Geometry check sheet. Reference: the model listing, model coordinates, mm. A direction names the side the tool comes from. Give positions to 0.01 mm unless a question says otherwise; leave off trailing zeros. Write each loop counter-clockwise with the first axis right and the second up, starting at its lowest first coordinate (ties: lowest second). Pieces come first, ordered by that corner, then holes. Notation, with made-up numbers: (12, 26.25) -> (42, 26.25) arc R20 cw to (42, 35.25) -> close; hole circle Ø4 at (-7, 3). An arc over 180 degrees is marked (long way). Use a Markdown table: item, result. Add a question column.
from build123d import *

# Parameters (mm, degrees)
SKETCH_1_R          = 3
EXTRUDE_1_DEPTH     = 18
CHAMFER_1_SIZE      = 0.5
CUT_EXTRUDE_1_DEPTH = 12


with BuildPart() as part:
    # Эскиз1 → Бобышка-Вытянуть1 (new body)
    with BuildSketch(Plane(origin=(0, 0, 0), x_dir=(1, 0, 0), z_dir=(0, 1, 0))):
        Circle(SKETCH_1_R)
    extrude(amount=EXTRUDE_1_DEPTH)

    # Фаска1
    chamfer_1_edges = [part.edges().sort_by_distance(p)[0] for p in [
        (-3, 18, 0),
    ]]
    chamfer(chamfer_1_edges, length=CHAMFER_1_SIZE)

    # Эскиз2 → Вырез-Вытянуть1 (cut)
    with BuildSketch(Plane(origin=(0, 18, 0), x_dir=(1, 0, 0), z_dir=(0, 1, 0))):
        with BuildLine():
            Line((-2.4, 1.8), (2.4, 1.8))
            ThreePointArc((2.4, 1.8), (0, 3), (-2.4, 1.8))
        make_face()
    extrude(amount=-CUT_EXTRUDE_1_DEPTH, mode=Mode.SUBTRACT)


solid = part.part
1) Sectioned sample at A-A, the plane x = 0. Enter the section's corners in (y, z), and give its area (3 significant figures).
2) Sectioned sample at D-D, the plane y = 8.5. Enter the section's corners in (x, z).
3) Sectioned sample at C-C, the plane z = -2.45. Enter the section's corners in (x, y), and give its area (3 significant figures).
4) Tool access check on faces 1 (the face through (0, 12, -1.8)), 2 (the face through (0, 0, 0)). Record the directions out of +Z, -Z, +X, -X, +Y, -Y that give a thin tool (end or side, any length) a straight path to the whole face; none if there is none.
5) Gauge pin test, flat ends, axial feed: P1, Ø1, axis at x = 0.5, y = 7.5, coming from the -Z side; P2, Ø0.6, axis at x = -1, z = -2.5, coming from the +Y side; P3, Ø2, axis at y = 6, z = 2.5, coming from the +X side. Record the tip position at first contact, or that the pin passes through.
6) Sectioned sample at B-B, the plane y = 2.25. Enter the section's corners in (x, z).
7) Material ranges on probe 1 along X at (y, z) = (8.75, 1.8); probe 2 along X at (y, z) = (13, -0.15); probe 3 along Y at (x, z) = (-2.2, -2), recorded low to high. Write a range as [from, to].
Check values:
| question | item | result |
|---|---|---|
| 1 | outline | (0, -3) -> (6, -3) -> (6, -1.8) -> (18, -1.8) -> (18, 2.5) -> (17.5, 3) -> (0, 3) -> close |
| 1 | area | 93.5 mm² |
| 2 | outline | (-2.4, -1.8) -> (2.4, -1.8) arc R3 ccw (long way) to start |
| 3 | outline | (-1.73, 0) -> (1.73, 0) -> (1.73, 6) -> (-1.73, 6) -> close |
| 3 | area | 20.8 mm² |
| 4 | face 1 | -Z, +X, -X, +Y |
| 4 | face 2 | +Z, -Z, +X, -X, -Y |
| 5 | P1 | z = -1.8 |
| 5 | P2 | y = 6 |
| 5 | P3 | x = 2.6 |
| 6 | outline | circle Ø6 at (0, 0) |
| 7 | probe 1 | [-2.4, 2.4] |
| 7 | probe 2 | [-3, 3] |
| 7 | probe 3 | [0, 6] |
